Build history of the part. All positions in model axes, mm. A direction names the side the tool comes from. Round coordinates to 2 decimals unless told otherwise and drop trailing zeros. Loops run counter-clockwise (first coordinate to the right, second up) from the corner with the lowest first, then second, coordinate; pieces in that order, holes last. Notation, with made-up numbers: (78, -33) - (83, -33) arc R17 cw to (83, -4) - close; hole circle Ø2 at (-2, 18.25). An arc over 180 degrees is marked (long way). Use one line per item in the form item = value. Start each with the question number.
Q1. 3-axis set-ups, long thin cutter, end or side, ignore diameter. For faces 1 (the face through (0, -4, 20)), 2 (the face through (6, -4, 50)), 3 (the face through (-17, 0, 21)), 4 (the face through (-35, -4, -4)): which of +Z, -Z, +X, -X, +Y, -Y reach the whole face in a straight line?
Q2. Pin check, flat tips, straight feed: pin 1 (2.5 mm diameter, centred on y = -2, z = 61, fed in from +X); pin 2 (1 mm diameter, centred on y = -2, z = 59, fed in from -X); pin 3 (1 mm diameter, centred on x = -19, y = -3.5, fed in from +Z). Stop position of each tip, or through.
Q3. Saw through at C-C (x = -9). Give the cut face in (y, z), then the cut area to 3 significant figures.
Q4. Saw through at A-A (y = -5.5). Give the cut face in (x, z), then the cut area to 3 significant figures.
Q5. Drill centre lines: line 1 (X direction, y = -0.25, z = -5); line 2 (Z direction, x = -2, y = -7); line 3 (Z direction, x = -47, y = -6.75). Where is each one in solid material? Low to high.
Q6. Saw through at B-B (z = 21). Give the cut face in (x, y).
```python
from build123d import *

# Parameters (mm, degrees)
F1_DEPTH = 8


with BuildPart() as f1:
    # F0 (on Front) → F1 (new body)
    with BuildSketch(Plane.XZ):
        with BuildLine():
            ThreePointArc((-57.197906, 8.402255), (-58.117129, 3.00141), (-53.533938, 0))
            Line((-53.533938, 0), (-35, 0))
            Line((-35, 0), (-35, -9))
            Line((-35, -9), (-20, -9))
            Line((-20, -9), (-20, 0))
            Line((-20, 0), (-10, 0))
            ThreePointArc((-10, 0), (-2.928932, 2.928932), (0, 10))
            Line((0, 10), (0, 30))
            Line((0, 30), (11, 30))
            Line((11, 30), (11, 50))
            Line((11, 50), (0, 50))
            Line((0, 50), (0, 64.906927))
            ThreePointArc((0, 64.906927), (-1.268964, 66.768536), (-3.465587, 66.267829))
            Line((-3.465587, 66.267829), (-57.197906, 8.402255))
        make_face()
    extrude(amount=F1_DEPTH)


solid = f1.part
```
Report:
q1.face_1 = -Z, +X, +Y, -Y
q1.face_2 = +Z, +X, +Y, -Y
q1.face_3 = +Z, -Z, +X, -X, +Y
q1.face_4 = -Z, -X, +Y, -Y
q2.pin_1 = 0
q2.pin_2 = -10.68
q2.pin_3 = 50.08
q3.outline = (-8, 0.05) - (0, 0.05) - (0, 60.31) - (-8, 60.31) - close
q3.area = 482 mm²
q4.outline = (-57.2, 8.4) arc R5 ccw to (-53.53, 0) - (-35, 0) - (-35, -9) - (-20, -9) - (-20, 0) - (-10, 0) arc R10 ccw to (0, 10) - (0, 30) - (11, 30) - (11, 50) - (0, 50) - (0, 64.91) arc R2 ccw to (-3.47, 66.27) - close
q4.area = 2,570 mm²
q5.line_1 = -35 to -20
q5.line_2 = 4 to 66.91
q5.line_3 = 0 to 19.38
q6.outline = (-45.5, -8) - (0, -8) - (0, 0) - (-45.5, 0) - close
